Autodesk Fusion 360 part; units mm, degrees
sketch "Skizze1" plane through (0, 0, 0) normal (0, 0, 1) x (1, 0, 0)
  line L0 (0, 0) -> (65, 0)
  line L1 (65, 0) -> (65, 56)
  line L2 (65, 56) -> (0, 56)
  line L3 (0, 56) -> (0, 0)
  circle A0 centre (61.5, 52.5) radius 1.5
  circle A1 centre (3.5, 52.5) radius 1.5
  circle A2 centre (3.5, 3.5) radius 1.5
  circle A3 centre (61.5, 3.5) radius 1.5
  line L4 (3.5, 3.5) -> (61.5, 3.5) construction
  line L5 (61.5, 3.5) -> (61.5, 52.5) construction
  line L6 (61.5, 52.5) -> (3.5, 52.5) construction
  line L7 (3.5, 52.5) -> (3.5, 3.5) construction
  line L8 (9.5, 39.8) -> (56.2, 39.8) construction
  line L9 (56.2, 39.8) -> (56.2, 23.3) construction
  line L10 (56.2, 23.3) -> (9.5, 23.3) construction
  line L11 (9.5, 23.3) -> (9.5, 39.8) construction
  line L12 (18.5, 39.8) -> (18.5, 35.3) construction
  line L13 (18.5, 35.3) -> (9.5, 35.3) construction
  line L14 (19.5, 25) -> (33.5, 25) construction
  line L15 (33.5, 25) -> (33.5, 39) construction
  line L16 (33.5, 39) -> (19.5, 39) construction
  line L17 (19.5, 39) -> (19.5, 25) construction
  line L18 (7, 49.3) -> (17.5, 49.3) construction
  line L19 (17.5, 49.3) -> (17.5, 36.3) construction
  line L20 (17.5, 36.3) -> (7, 36.3) construction
  line L21 (7, 36.3) -> (7, 49.3) construction
  line L22 (52.2, 39.8) -> (52.2, 23.3) construction
  line L23 (17.5, 23.3) -> (17.5, 36.3) construction
  circle A4 centre (3.5, 52.5) radius 3.1
  circle A5 centre (61.5, 52.5) radius 3.1
  circle A6 centre (3.5, 3.5) radius 3.1
  circle A7 centre (61.5, 3.5) radius 3.1
  line L24 (6.6, 52.5) -> (0.4, 52.5) construction
  line L25 (0.4, 52.5) -> (0.4, 40.5)
  line L26 (0.4, 40.5) -> (6.6, 40.5)
  line L27 (6.6, 40.5) -> (6.6, 52.5)
  line L28 (61.5, 49.4) -> (68, 49.4)
  line L29 (68, 49.4) -> (68, 55.6)
  line L30 (68, 55.6) -> (61.5, 55.6)
  line L31 (61.5, 55.6) -> (61.5, 49.4) construction
  dimension "d1" = 65
  dimension "d2" = 56
  dimension "d3" = 49
  dimension "d4" = 3.5
  dimension "d5" = 4
  dimension "d6" = 3.5
  dimension "d7" = 3.5
  dimension "d8" = 3
  dimension "d9" = 3
  dimension "d10" = 3
  dimension "d11" = 3
  dimension "d12" = 46.7
  dimension "d13" = 16.5
  dimension "d14" = 4.5
  dimension "d15" = 9
  dimension "d16" = 14
  dimension "d17" = 14
  dimension "d18" = 17
  dimension "d19" = 19.5
  dimension "d20" = 10.5
  dimension "d21" = 13
  dimension "d22" = 6.7
  dimension "d23" = 7
  dimension "d24" = 2
  dimension "d25" = 1
  dimension "d26" = 1
  dimension "d27" = 1
  dimension "d28" = 4
  dimension "d29" = 8
  dimension "d30" = 6.2
  dimension "d31" = 6.2
  dimension "d32" = 6.2
  dimension "d33" = 6.2
  dimension "d36" = 12
  dimension "d37" = 6.5
ref_plane "Arbeitsebene1" through (0, 0, 4) normal (0, 0, 1) x (1, 0, 0)
sketch "Skizze2" plane through (0, 0, 4) normal (0, 0, 1) x (1, 0, 0)
  line L0 (52.2, 39.8) -> (52.2, 23.3)
  line L1 (56.2, 39.8) -> (56.2, 23.3)
  line L2 (56.2, 23.3) -> (9.5, 23.3)
  line L3 (9.5, 39.8) -> (56.2, 39.8)
  line L4 (9.5, 23.3) -> (9.5, 39.8)
  line L5 (17.5, 23.3) -> (17.5, 36.3)
  line L6 (17.5, 49.3) -> (17.5, 36.3)
  line L7 (56.2, 39.8) -> (9.5, 39.8)
  line L8 (9.5, 39.8) -> (9.5, 47.8)
  line L9 (9.5, 47.8) -> (56.2, 47.8)
  line L10 (56.2, 47.8) -> (56.2, 39.8)
  line L11 (56.2, 47.8) -> (68, 47.8)
  line L12 (68, 47.8) -> (68, 15)
  line L13 (68, 15) -> (56.2, 15)
  line L14 (56.2, 15) -> (56.2, 47.8)
  line L15 (0, 0) -> (65, 0)
  line L16 (68, 49.4) -> (68, 55.6)
  line L17 (68, 15) -> (63, 15)
  line L18 (63, 15) -> (63, 20)
  line L19 (63, 20) -> (68, 20)
  line L20 (68, 20) -> (68, 15)
  line L21 (68, 49.4) -> (68, 47.8)
  line L22 (61.5, 49.4) -> (68, 49.4)
  line L23 (65, 0) -> (65, 56)
  line L24 (65, 47.8) -> (65, 49.4)
  line L25 (58.4, 47.8) -> (64.6, 47.8)
  line L26 (64.6, 47.8) -> (64.6, 43.5)
  line L27 (64.6, 43.5) -> (58.4, 43.5)
  line L28 (58.4, 43.5) -> (58.4, 47.8)
  circle A0 centre (61.5, 52.5) radius 3.1
  line L29 (58.4, 15) -> (64.6, 15)
  line L30 (64.6, 15) -> (64.6, 3.5)
  line L31 (64.6, 3.5) -> (58.4, 3.5)
  line L32 (58.4, 3.5) -> (58.4, 15)
  circle A1 centre (61.5, 3.5) radius 3.1
  line L33 (6.6, 40.5) -> (9.5, 40.5)
  line L34 (6.6, 40.5) -> (6.6, 52.5)
  line L35 (9.5, 47.8) -> (6.6, 47.8)
  line L36 (6.6, 3.5) -> (0.4, 3.5)
  line L37 (0.4, 3.5) -> (0.4, 15.5)
  line L38 (0.4, 15.5) -> (6.6, 15.5)
  line L39 (6.6, 15.5) -> (6.6, 3.5)
  circle A2 centre (3.5, 3.5) radius 3.1
  line L40 (3.5, 3.5) -> (61.5, 3.5)
  line L41 (6.6, 40.5) -> (6.6, 15.5)
  line L42 (9.5, 23.3) -> (9.5, 6.6)
  line L43 (6.6, 6.6) -> (9.5, 6.6)
  line L44 (6.6, 36.3) -> (9.5, 36.3)
  dimension "d45" = 8
  dimension "d50" = 15
  dimension "d52" = 20
  dimension "d53" = 5
  dimension "d70" = 9
  dimension "d81" = 12
extrude "Extrusion3" add sketch "Skizze2" along normal blind 2 contours L0 L1 L2 L3 L7 L14 | L2 L3 L4 L5 L6 L7 makes body 1 at (54.8667, 28.8, 4) makes body 2 at (12.1667, 28.8, 4)
chamfer "Fase1" distance 2 angle 45 1 edges at (17.5, 31.55, 6) measured on face at (12.1667, 28.8, 6) on bodies 2
extrude "Extrusion4" add sketch "Skizze2" along normal blind 2 contours L3 L6 L7 L9 L10 L14 | L3 L6 L7 L8 L9 bodies 1 2
extrude "Extrusion5" add sketch "Skizze2" against normal blind 3 contours L3 L6 L7 L9 L10 L14 bodies 1
extrude "Extrusion6" add sketch "Skizze2" along normal blind 2 and the other way blind 2.4 contours L1 L10 L11 L13 L14 L18 L19 L23 L26 L27 L28 L29 | L11 L12 L19 L23 bodies 1
extrude "Extrusion7" add sketch "Skizze1" along normal blind 6 separate body contours L1 A5 L28 L30 | L1 L28 L29 L30 | A5 makes body 3
extrude "Extrusion8" add sketch "Skizze1" along normal blind 6 separate body contours A4 | A4 L25 L26 L27 makes body 4
extrude "Extrusion9" add sketch "Skizze1" along normal blind 6 separate body contours A7 makes body 5
extrude "Extrusion10" add sketch "Skizze1" along normal blind 6 separate body contours A6 makes body 6
extrude "Extrusion11" add sketch "Skizze2" along normal blind 2 and the other way blind 2.4 contours L11 L21 L22 L23 L24 bodies 1 3
extrude "Extrusion12" add sketch "Skizze2" along normal blind 2 and the other way blind 2.4 contours L13 L17 L29 L30 L32 A1 bodies 1 5
extrude "Extrusion13" add sketch "Skizze2" against normal blind 1.7 contours L3 L6 L7 L8 L9 bodies 1
extrude "Extrusion14" add sketch "Skizze2" along normal blind 2 contours L8 L33 L34 L35 bodies 1 4
extrude "Extrusion15" add sketch "Skizze2" against normal blind 1.7 contours L8 L33 L34 L35 bodies 1
extrude "Extrusion16" add sketch "Skizze2" against normal blind 1.7 separate body contours L4 L8 L33 L41 L44 makes body 7
extrude "Extrusion17" add sketch "Skizze2" against normal blind 2.4 contours L4 L39 L41 L42 L43 L44 | L37 L38 L39 A2 bodies 6 1 7
extrude "Extrusion18" add sketch "Skizze2" along normal blind 2 contours L4 L8 L33 L41 L44 | L4 L39 L41 L42 L43 L44 | L37 L38 L39 A2 bodies 6
equation "d6 = d4"
equation "d7 = d4"
equation "d9 = d8"
equation "d10 = d8"
equation "d11 = d8"
Input: part model. Units: mm. Frame: model coordinates. A direction names the side the tool comes from. Coordinates: 2 decimals unless noted, no trailing zeros. Loops run counter-clockwise (first coordinate to the right, second up) from the corner with the lowest first, then second, coordinate; pieces in that order, holes last.
(1) Section C-C on z = 3.1. Count the separate pieces of the cut face and the enclosed holes in it, then the cut area to 3 significant figures.
(2) Material intervals for probe 1 along Y at (x, z) = (3.5, 4.7); probe 2 along X at (y, z) = (7, 4.8); probe 3 along Y at (x, z) = (61.5, 1.35), sorted ascending.
(3) Section D-D on y = 13. Return the cut outline in (x, z).
(4) Set-up query: faces 1 (the face through (61.096, 0.426, 2.291)), 2 (the face through (56.2, 25, 3)), 3 (the face through (3, 40.5, 3)). Return all of +Z, -Z, +X, -X, +Y, -Y with unobstructed straight access to the full face (end or side cutting, diameter ignored); none if empty.
(5) Section B-B on x = 3.5. Return the cut outline in (y, z).
(6) Pull-direction query (Y, two-part tool) for faces 4 (the face through (64.6, 46, 4)), 5 (the face through (54, 32, 4)), 6 (the face through (8, 6.6, 4)); classes: released by +Y, released by -Y, zero draft, split by the parting line, or undercut.
(7) First-contact query: pin 1 Ø3 at (x, y) = (55, 29.5) entering from -Z; pin 2 Ø5 at (x, y) = (21, 48.5) entering from -Z; pin 3 Ø0.6 at (x, z) = (14.5, 5.5) entering from -Y; pin 4 Ø1.8 at (x, y) = (3.5, 3.5) entering from +Z. Flat tips, straight axial feed; report the tip coordinate or a pass-through.
Data:
1. separate pieces: 1
1. enclosed holes: 4
1. area: 1,130 mm2
2. probe 1: y = 0.4 to 2, 5 to 15.5, 40.5 to 51, 54 to 55.6
2. probe 2: x = 0.4 to 9.5, 58.4 to 64.6
2. probe 3: y = 0.4 to 2, 5 to 6.6, 49.4 to 51, 54 to 55.6
3. outline: (0.4, 1.6) - (9.5, 1.6) - (9.5, 6) - (0.4, 6) - close; (58.4, 1.6) - (64.6, 1.6) - (64.6, 6) - (58.4, 6) - close
4. face 1: -Z
4. face 2: -Z, -Y
4. face 3: +Z, -Z, -X
5. outline: (0.4, 0) - (2, 0) - (2, 6) - (0.4, 6) - close; (5, 0) - (6.6, 0) - (6.6, 1.6) - (15.5, 1.6) - (15.5, 6) - (5, 6) - close; (40.5, 0) - (51, 0) - (51, 6) - (40.5, 6) - close; (54, 0) - (55.6, 0) - (55.6, 6) - (54, 6) - close
6. face 4: undercut
6. face 5: zero draft
6. face 6: released by -Y
7. pin 1: stops at z = 1.6
7. pin 2: stops at z = 1
7. pin 3: stops at y = 23.3
7. pin 4: passes through
